from build123d import *

# Parameters (mm, degrees)
SALIENTE_EXTRUIR1_DEPTH = 20


with BuildPart() as part:
    # Croquis1 → Saliente-Extruir1 (new body)
    with BuildSketch(Plane.XY):
        with BuildLine():
            Line((853.07011629, 88.169264479), (931.851074637, 177.517253669))
            Line((931.851074637, 177.517253669), (1123.432307328, 459.574764509))
            Line((1123.432307328, 459.574764509), (1144.834105581, 519.888923222))
            Line((1144.834105581, 519.888923222), (1152.616577673, 568.529373797))
            Line((1152.616577673, 568.529373797), (1148.725341627, 619.115442395))
            Line((1148.725341627, 619.115442395), (1134.133206454, 654.13656681))
            Line((1134.133206454, 654.13656681), (1112.467017385, 668.852839378))
            Line((1112.467017385, 668.852839378), (1089.383991925, 668.852839378))
            Line((1089.383991925, 668.852839378), (1060.811863494, 656.947785866))
            Line((1060.811863494, 656.947785866), (1035.115093442, 619.115442395))
            Line((1035.115093442, 619.115442395), (1015.768853134, 590.989004825))
            Line((1015.768853134, 590.989004825), (762.554169484, 303.810182778))
            Line((762.554169484, 303.810182778), (506.078323887, 244.468113377))
            ThreePointArc((506.078323887, 244.468113377), (371.222836086, 109.612625576), (506.078323887, -25.242862225))
            Line((506.078323887, -25.242862225), (853.07011629, 88.169264479))
        make_face()
    extrude(amount=SALIENTE_EXTRUIR1_DEPTH)


solid = part.part
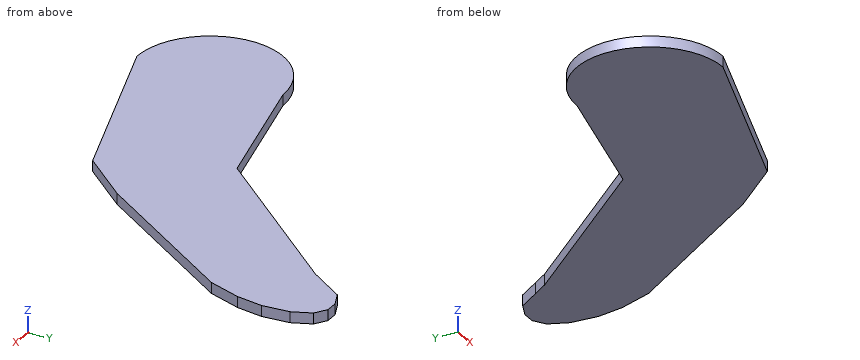
Input: part model. Units: mm. Frame: model coordinates. Coordinates: 2 decimals unless noted, no trailing zeros. Loops run counter-clockwise (first coordinate to the right, second up) from the corner with the lowest first, then second, coordinate; pieces in that order, holes last. Notation, with made-up numbers: (-34, -35) -> (-2, -35) arc R22 ccw to (-2, -7) -> close; hole circle Ø10 at (61, 84). An arc over 180 degrees is marked (long way). Write item = value, one per line. Start each with the question number.
Item 1: First-contact query: P1, Ø2, axis at y = 384, z = 9, coming from the +X side; P2, Ø1, axis at x = 759, z = 9.5, coming from the +Y side; P3, Ø12, axis at y = 387.5, z = 10, coming from the +X side. Flat tips, straight axial feed; report the tip coordinate or a pass-through.
Item 2: Cut plane A-A, the plane z = 13.5. Return loops of the section in (x, y).
Item 3: Cut plane C-C, the plane x = 1078.5. Return loops of the section in (y, z), plus the area to 3 significant figures.
Item 4: Cut plane B-B, the plane y = 377. Return loops of the section in (x, z), plus the area to 3 significant figures.
Item 5: Material intervals for line 1 (X direction, y = 417, z = 7.75); line 2 (Y direction, x = 917, z = 18.5); line 3 (Y direction, x = 839.5, z = 13), sorted ascending.
Ans:
q1.P1 = 1072.78
q1.P2 = 303.1
q1.P3 = 1078.55
q2.outline = (506.08, -25.24) -> (853.07, 88.17) -> (931.85, 177.52) -> (1123.43, 459.57) -> (1144.83, 519.89) -> (1152.62, 568.53) -> (1148.73, 619.12) -> (1134.13, 654.14) -> (1112.47, 668.85) -> (1089.38, 668.85) -> (1060.81, 656.95) -> (1035.12, 619.12) -> (1015.77, 590.99) -> (762.55, 303.81) -> (506.08, 244.47) arc R134.86 ccw to start
q3.outline = (393.42, 0) -> (664.32, 0) -> (664.32, 20) -> (393.42, 20) -> close
q3.area = 5,420 mm²
q4.outline = (827.09, 0) -> (1067.35, 0) -> (1067.35, 20) -> (827.09, 20) -> close
q4.area = 4,810 mm²
q5.line_1 = 862.36 to 1094.51
q5.line_2 = 160.67 to 478.97
q5.line_3 = 83.73 to 391.08
